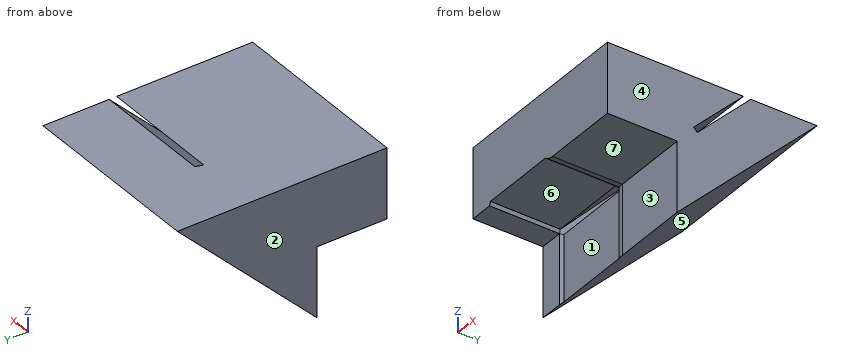
```python
from build123d import *

# Parameters (mm, degrees)
SKETCH1_W           = 50
SKETCH1_H           = 20
BOSS_EXTRUDE1_DEPTH = 10
CUT_EXTRUDE1_DEPTH  = 0.375
BOSS_EXTRUDE3_DEPTH = 10
BOSS_EXTRUDE4_DEPTH = 10
SKETCH5_W           = 25.687022838
SKETCH5_H           = 30.894675689
CUT_EXTRUDE3_DEPTH  = 41.311288741
CUT_EXTRUDE4_DEPTH  = 36.057096286
FILLET1_R           = 2
FILLET2_R           = 2


with BuildPart() as part:
    # Sketch1 → Boss-Extrude1 (new body)
    with BuildSketch(Plane.XY):
        Rectangle(SKETCH1_W, SKETCH1_H)
    extrude(amount=BOSS_EXTRUDE1_DEPTH)

    # Sketch2 → Cut-Extrude1 (cut, symmetric)
    with BuildSketch(Plane(origin=(0, -5, 5), x_dir=(1, 0, 0), z_dir=(0, -0.7071067811865464, 0.7071067811865488))):
        Polygon((-23, -10.071067812), (35.375550351, 5.570613762), (29.163893269, 28.752833593), (-10.439065609, 18.141252744), align=None)
    extrude(amount=CUT_EXTRUDE1_DEPTH, both=True, mode=Mode.SUBTRACT)

    # Sketch3 → Boss-Extrude3 (add)
    with BuildSketch(Plane.XZ.offset(10)):
        Polygon((-25, 0), (-21.664313944, 0), (-21.497353187, 0.530330086), (-10.404328524, 0.530330086), (-11.803847577, 0), (25, 0), (25, 10), (-25, 10), align=None)
    extrude(amount=BOSS_EXTRUDE3_DEPTH)

    # Sketch4 → Boss-Extrude4 (add)
    with BuildSketch(Plane(origin=(0, 0, 0), x_dir=(-1, 0, 0), z_dir=(0, 0, -1))):
        Polygon((10.404328524, -9.469669914), (21.497353187, -9.469669914), (21.664313944, -10), (25, -10), (25, 10), (-25, 10), (-25, -10), (11.803847577, -10), align=None)
    extrude(amount=BOSS_EXTRUDE4_DEPTH)

    # Sketch5 → Cut-Extrude3 (cut, through all)
    with BuildSketch(Plane.XZ.offset(20)):
        with Locations((14.843511419, 0.908787841)):
            Rectangle(SKETCH5_W, SKETCH5_H)
    extrude(amount=-CUT_EXTRUDE3_DEPTH, mode=Mode.SUBTRACT)

    # Sketch6 → Cut-Extrude4 (cut, through all)
    with BuildSketch(Plane(origin=(2, 0, 0), x_dir=(0, 0, -1), z_dir=(1, 0, 0))):
        Polygon((-10, 10), (10, -10), (10, 10), align=None)
    extrude(amount=-CUT_EXTRUDE4_DEPTH, mode=Mode.SUBTRACT)

    # Fillet1
    # the kernel refuses this fillet: 2 mm, written as the material it takes off along each edge
    with BuildSketch(Plane(origin=(-11.803847577, -10, 0), x_dir=(1, 0, 0), z_dir=(0, 0, -1))) as fillet1_piece_1:
        with BuildLine():
            CenterArc((2.756010978, -2), FILLET1_R, 90, 42.706727968)
            Line((1.399519053, -0.530330086), (0, 0))
            Line((0, 0), (2.756010978, 0))
        make_face()
    extrude(amount=16.890027445, mode=Mode.SUBTRACT)

    # Fillet2
    # the kernel refuses this fillet: 2 mm, written as the material it takes off along each edge
    with BuildSketch(Plane(origin=(-11.803847577, -3.109972555, 0), x_dir=(1, 0, 0), z_dir=(0, -1, 0))) as fillet2_piece_1_section:
        with BuildLine():
            CenterArc((2.756010978, 2), FILLET2_R, 227.293272032, 42.706727968)
            Line((1.399519053, 0.530330086), (0, 0))
            Line((0, 0), (2.756010978, 0))
        make_face()
    fillet2_piece_1 = extrude(amount=23.780054891, mode=Mode.PRIVATE)
    fillet2_piece_1 = split(fillet2_piece_1, bisect_by=Plane(origin=(-9.777530732, -9.469669914, 0.133569591), z_dir=(0, -1, 0)), keep=Keep.TOP, mode=Mode.PRIVATE)
    fillet2_piece_1 = fillet2_piece_1 - Plane(origin=(-9.047836599, -8, 0.133569591), x_dir=(1, 0, 0), z_dir=(0, 0, 1)) * Cylinder(2, 59, mode=Mode.PRIVATE)
    add(fillet2_piece_1, mode=Mode.SUBTRACT)


solid = part.part
```
Source: CAD feature listing. Evaluate the final solid. Frame: model axes, mm. Face numbers are marked on the shaded views. A direction names the side the tool comes from. Give positions to 0.01 mm unless a question says otherwise; leave off trailing zeros. Write each loop counter-clockwise with the first axis right and the second up, starting at its lowest first coordinate (ties: lowest second). Pieces come first, ordered by that corner, then holes. Notation, with made-up numbers: (78.5, 84) - (126.5, 84) arc R20 ccw to (126.5, 112) - close; hole circle Ø8 at (74.25, -18.75). An arc over 180 degrees is marked (long way). One line per item, written item: value. Start each with the question number.
Q1. Section query C-C, the plane x = -8. Return the cut outline in (y, z).
Q2. Section query B-B, the plane y = -17.25. Return the cut outline in (x, z), then the cut area to 3 significant figures.
Q3. First-contact query: pin 1 Ø8 at (x, y) = (-8.5, 5) entering from -Z; pin 2 Ø1 at (x, y) = (-24, -15.5) entering from -Z; pin 3 Ø3 at (x, z) = (-13.5, -4) entering from -Y. Flat tips, straight axial feed; report the tip coordinate or a pass-through.
Q4. Section query D-D, the plane x = -23. Return the cut outline in (y, z), then the cut area to 3 significant figures.
Q5. Draft query along X for the marked faces 1, 2, 3 and 4. Return one class per face: +X half, -X half, draft (parallel to the pull), parting line (faces both ways), or undercut.
Q6. Material intervals for probe 1 along Z at (x, y) = (-5.75, -13); probe 2 along Y at (x, z) = (-1.25, 4.5); probe 3 along Y at (x, z) = (-8.25, 7.75), sorted ascending. Write a range as from..to.
Q7. Section query A-A, the plane z = -5.75. Return the cut outline in (x, y), then the cut area to 3 significant figures.
Q8. Set-up query: the marked faces 5, 6 and 7. Return all of +Z, -Z, +X, -X, +Y, -Y with unobstructed straight access to the full face (end or side cutting, diameter ignored); none if empty.
Answer:
1. outline: (-20, 0) - (-10, 0) - (-10, -10) - (10, 10) - (0.53, 10) - (-9.01, 0.46) - (-9.54, 0.99) - (-0.53, 10) - (-20, 10) - close
2. outline: (-25, 0) - (-21.66, 0) - (-21.5, 0.53) - (-10.4, 0.53) arc R2 ccw to (-9.05, 0) - (2, 0) - (2, 10) - (-25, 10) - close
2. area: 264 mm2
3. pin 1: stops at z = 1
3. pin 2: stops at z = 0
3. pin 3: stops at y = -9.47
4. outline: (-20, 0) - (-10, 0) - (-10, -10) - (10, 10) - (-20, 10) - close
4. area: 300 mm2
5. face 1: undercut
5. face 2: -X half
5. face 3: draft
5. face 4: +X half
6. probe 1: z = 0..10
6. probe 2: y = -20..-6.03, -4.97..4.5
6. probe 3: y = -20..-2.78, -1.72..7.75
7. outline: (-25, -10) - (-21.66, -10) - (-21.5, -9.47) - (-10.4, -9.47) arc R2 ccw to (-9.05, -10) - (2, -10) - (2, -5.75) - (-25, -5.75) - close
7. area: 109 mm2
8. face 5: -Z, +X, -X, +Y
8. face 6: -Z, -Y
8. face 7: -Z, +X, -X, -Y
